```python
from build123d import *

# Parameters (mm, degrees)
F0_W         = 82.2881497443
F0_H         = 82.288146019
F0_R         = 4.2853217598
F1_DEPTH     = 25.4
F2_T1_DEPTH  = 33.02
F2_T3_DEPTH  = 107.688146019
F2_T5_DEPTH  = 72.128146019
F2_T7_DEPTH  = 72.1281497443
F2_S11_W     = 5.08
F2_S11_H     = 5.08
F2_T12_DEPTH = 5.08
F2_S17_W     = 5.08
F2_S17_H     = 5.08
F2_T18_DEPTH = 5.08
F2_S23_W     = 5.08
F2_S23_H     = 5.08
F2_T24_DEPTH = 5.08
F2_S29_W     = 5.08
F2_S29_H     = 5.08
F2_T30_DEPTH = 5.08


# Not quite as in the source:
# - a fillet or chamfer that OpenCascade refuses, or shapes differently, is made with other operations: its cross-section is extruded or revolved along the edge and cut away or added
# - a feature of the source that left no trace in its solid (it failed there, or was rolled back) is left out


with BuildPart() as f1:
    # F0 (on Front) → F1 (new body)
    with BuildSketch(Plane.XZ):
        with Locations((2.3490097374, -1.9460879266)):
            Rectangle(F0_W, F0_H)
        with Locations((-30.2557293326, 28.0709732324)):
            Circle(F0_R, mode=Mode.SUBTRACT)
        with Locations((36.1182056367, 29.1060488671)):
            Circle(F0_R, mode=Mode.SUBTRACT)
    extrude(amount=F1_DEPTH)

    # F2: fillet of radius 5.08 on 12 edges, made by hand

    # F2_s2 → F2_t1 (cut)
    with BuildSketch(Plane.XZ.offset(-12.7)):
        with BuildLine():
            ThreePointArc((38.4130846095, -43.0901609361), (42.0051870579, -41.6022633845), (43.4930846095, -38.0101609361))
            Line((43.4930846095, -38.0101609361), (43.4930846095, -43.0901609361))
            Line((43.4930846095, -43.0901609361), (38.4130846095, -43.0901609361))
        make_face()
        with BuildLine():
            ThreePointArc((38.4130846095, 39.1979850829), (42.0051870579, 37.7100875313), (43.4930846095, 34.1179850829))
            Line((43.4930846095, 34.1179850829), (43.4930846095, 39.1979850829))
            Line((43.4930846095, 39.1979850829), (38.4130846095, 39.1979850829))
        make_face()
        with BuildLine():
            ThreePointArc((-33.7150651348, 39.1979850829), (-37.3071675832, 37.7100875313), (-38.7950651348, 34.1179850829))
            Line((-38.7950651348, 34.1179850829), (-38.7950651348, 39.1979850829))
            Line((-38.7950651348, 39.1979850829), (-33.7150651348, 39.1979850829))
        make_face()
        with BuildLine():
            ThreePointArc((-38.7950651348, -38.0101609361), (-37.3071675832, -41.6022633845), (-33.7150651348, -43.0901609361))
            Line((-33.7150651348, -43.0901609361), (-38.7950651348, -43.0901609361))
            Line((-38.7950651348, -43.0901609361), (-38.7950651348, -38.0101609361))
        make_face()
    extrude(amount=F2_T1_DEPTH, mode=Mode.SUBTRACT)

    # F2_s4 → F2_t3 (cut)
    with BuildSketch(Plane.XY.offset(-55.7901609361)):
        with BuildLine():
            ThreePointArc((43.4930846095, -5.08), (42.0051870579, -1.4878975516), (38.4130846095, 0))
            Line((38.4130846095, 0), (43.4930846095, 0))
            Line((43.4930846095, 0), (43.4930846095, -5.08))
        make_face()
        with BuildLine():
            ThreePointArc((-38.7950651348, -5.08), (-37.3071675832, -1.4878975516), (-33.7150651348, 0))
            Line((-33.7150651348, 0), (-38.7950651348, 0))
            Line((-38.7950651348, 0), (-38.7950651348, -5.08))
        make_face()
    extrude(amount=F2_T3_DEPTH, mode=Mode.SUBTRACT)

    # F2_s6 → F2_t5 (cut)
    with BuildSketch(Plane.XY.offset(-38.0101609361)):
        with BuildLine():
            ThreePointArc((43.4930846095, -20.32), (42.0051870579, -23.9121024484), (38.4130846095, -25.4))
            Line((38.4130846095, -25.4), (43.4930846095, -25.4))
            Line((43.4930846095, -25.4), (43.4930846095, -20.32))
        make_face()
        with BuildLine():
            ThreePointArc((-38.7950651348, -20.32), (-37.3071675832, -23.9121024484), (-33.7150651348, -25.4))
            Line((-33.7150651348, -25.4), (-38.7950651348, -25.4))
            Line((-38.7950651348, -25.4), (-38.7950651348, -20.32))
        make_face()
    extrude(amount=F2_T5_DEPTH, mode=Mode.SUBTRACT)

    # F2_s8 → F2_t7 (cut)
    with BuildSketch(Plane.YZ.offset(-33.7150651348)):
        with BuildLine():
            ThreePointArc((-20.32, 39.1979850829), (-23.9121024484, 37.7100875313), (-25.4, 34.1179850829))
            Line((-25.4, 34.1179850829), (-25.4, 39.1979850829))
            Line((-25.4, 39.1979850829), (-20.32, 39.1979850829))
        make_face()
        with BuildLine():
            ThreePointArc((-20.32, -43.0901609361), (-23.9121024484, -41.6022633845), (-25.4, -38.0101609361))
            Line((-25.4, -38.0101609361), (-25.4, -43.0901609361))
            Line((-25.4, -43.0901609361), (-20.32, -43.0901609361))
        make_face()
    extrude(amount=F2_T7_DEPTH, mode=Mode.SUBTRACT)


with BuildPart() as f2_tool10:
    # F2_s11 → F2_t12 (new body)
    with BuildSketch(Plane.XY.offset(-38.0101609361)):
        with Locations((40.9530846095, -22.86)):
            Rectangle(F2_S11_W, F2_S11_H)
    extrude(amount=-F2_T12_DEPTH)

    # F2_s13 → F2_t14 (revolve, cut)
    with BuildSketch(Plane(origin=(38.4130846095, -20.32, -38.0101609361), x_dir=(-0.7071067812, 0.7071067812, 0), z_dir=(-0.7071067812, -0.7071067812, 0))):
        with BuildLine():
            ThreePointArc((0, -5.08), (5.08, 0), (0, 5.08))
            Line((0, 5.08), (0, -5.08))
        make_face()
    revolve(axis=Axis((38.4130846095, -20.32, -38.0101609361), (0, 0, -1)), mode=Mode.SUBTRACT)


with BuildPart() as f1_1:
    add(f1.part)

    # F2_t9: cut F2_tool10
    add(f2_tool10.part, mode=Mode.SUBTRACT)


with BuildPart() as f2_tool16:
    # F2_s17 → F2_t18 (new body)
    with BuildSketch(Plane.XY.offset(34.1179850829)):
        with Locations((40.9530846095, -22.86)):
            Rectangle(F2_S17_W, F2_S17_H)
    extrude(amount=F2_T18_DEPTH)

    # F2_s19 → F2_t20 (revolve, cut)
    with BuildSketch(Plane(origin=(38.4130846095, -20.32, 34.1179850829), x_dir=(-0.7071067812, 0.7071067812, 0), z_dir=(0.7071067812, 0.7071067812, 0))):
        with BuildLine():
            ThreePointArc((0, -5.08), (5.08, 0), (0, 5.08))
            Line((0, 5.08), (0, -5.08))
        make_face()
    revolve(axis=Axis((38.4130846095, -20.32, 34.1179850829), (0, 0, 1)), mode=Mode.SUBTRACT)


with BuildPart() as f1_2:
    add(f1_1.part)

    # F2_t15: cut F2_tool16
    add(f2_tool16.part, mode=Mode.SUBTRACT)


with BuildPart() as f2_tool22:
    # F2_s23 → F2_t24 (new body)
    with BuildSketch(Plane.XY.offset(34.1179850829)):
        with Locations((-36.2550651348, -22.86)):
            Rectangle(F2_S23_W, F2_S23_H)
    extrude(amount=F2_T24_DEPTH)

    # F2_s25 → F2_t26 (revolve, cut)
    with BuildSketch(Plane(origin=(-33.7150651348, -20.32, 34.1179850829), x_dir=(0.7071067812, 0.7071067812, 0), z_dir=(0.7071067812, -0.7071067812, 0))):
        with BuildLine():
            ThreePointArc((0, -5.08), (5.08, 0), (0, 5.08))
            Line((0, 5.08), (0, -5.08))
        make_face()
    revolve(axis=Axis((-33.7150651348, -20.32, 34.1179850829), (0, 0, 1)), mode=Mode.SUBTRACT)


with BuildPart() as f1_3:
    add(f1_2.part)

    # F2_t21: cut F2_tool22
    add(f2_tool22.part, mode=Mode.SUBTRACT)


with BuildPart() as f2_tool28:
    # F2_s29 → F2_t30 (new body)
    with BuildSketch(Plane.YZ.offset(-33.7150651348)):
        with Locations((-22.86, -40.5501609361)):
            Rectangle(F2_S29_W, F2_S29_H)
    extrude(amount=-F2_T30_DEPTH)

    # F2_s31 → F2_t32 (revolve, cut)
    with BuildSketch(Plane(origin=(-33.7150651348, -20.32, -38.0101609361), x_dir=(0, 0.7071067812, 0.7071067812), z_dir=(0, -0.7071067812, 0.7071067812))):
        with BuildLine():
            ThreePointArc((0, -5.08), (5.08, 0), (0, 5.08))
            Line((0, 5.08), (0, -5.08))
        make_face()
    revolve(axis=Axis((-33.7150651348, -20.32, -38.0101609361), (-1, 0, 0)), mode=Mode.SUBTRACT)


with BuildPart() as f1_4:
    add(f1_3.part)

    # F2_t27: cut F2_tool28
    add(f2_tool28.part, mode=Mode.SUBTRACT)

    # F2_s33 → F2_t34 (revolve, cut)
    with BuildSketch(Plane.XY.offset(28.0709732324)):
        with BuildLine():
            ThreePointArc((-25.9704075728, -20.32), (-24.4825100212, -23.9121024484), (-20.8904075728, -25.4))
            Line((-20.8904075728, -25.4), (-25.9704075728, -25.4))
            Line((-25.9704075728, -25.4), (-25.9704075728, -20.32))
        make_face()
    revolve(axis=Axis((-30.2557293326, -25.4, 28.0709732324), (0, -1, 0)), mode=Mode.SUBTRACT)

    # F2_s35 → F2_t36 (revolve, cut)
    with BuildSketch(Plane.XY.offset(29.1060488671)):
        with BuildLine():
            ThreePointArc((40.4035273965, -20.32), (41.8914249481, -23.9121024484), (45.4835273965, -25.4))
            Line((45.4835273965, -25.4), (40.4035273965, -25.4))
            Line((40.4035273965, -25.4), (40.4035273965, -20.32))
        make_face()
    revolve(axis=Axis((36.1182056367, -25.4, 29.1060488671), (0, -1, 0)), mode=Mode.SUBTRACT)


solid = f1_4.part
```
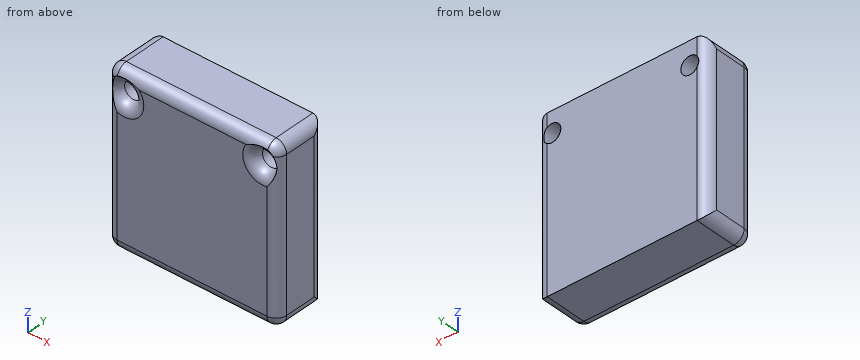
Work out the finished part from the listing and answer in its coordinate system (mm). Round coordinates to 2 decimals unless told otherwise and drop trailing zeros. Order: outer loops, then holes, each group sorted by start corner. A loop starts at its lowest first (then second) coordinate and runs counter-clockwise, first axis right, second up.
Q1. Find the intervals of material crossed by line 1 along X through (y, z) = (-13.25, 29); line 2 along X through (y, z) = (-7, 24.5); line 3 along X through (y, z) = (-5, -19.5), in increasing order.
Solution:
line 1: x = -38.8 to -34.44, -26.07 to 31.83, 40.4 to 43.49
line 2: x = -38.8 to -32.62, -27.89 to 43.49
line 3: x = -38.79 to 43.49
Q2. A cutting plane is placed at B-B, the plane y = -21.75. Determine the outline of the cut face in (x, z).
Solution:
outline: (-38.59, -38.01) arc R4.87 ccw to (-33.72, -42.88) - (38.41, -42.88) arc R4.87 ccw to (43.29, -38.01) - (43.29, 34.12) arc R4.87 ccw to (38.41, 38.99) - (-33.72, 38.99) arc R4.87 ccw to (-38.59, 34.12) - close; hole circle Ø8.98 at (-30.26, 28.07); hole circle Ø8.98 at (36.12, 29.11)
Q3. A cutting plane is placed at A-A, the plane y = -2. Determine the outline of the cut face in (x, z).
Solution:
outline: (-37.75, -41.09) arc R5.08 ccw to (-33.72, -43.09) - (38.41, -43.09) arc R5.08 ccw to (42.45, -41.09) - (42.45, 37.2) arc R5.08 ccw to (38.41, 39.2) - (-33.72, 39.2) arc R5.08 ccw to (-37.75, 37.2) - close; hole circle Ø8.57 at (-30.26, 28.07); hole circle Ø8.57 at (36.12, 29.11)
Q4. Given pin 1 Ø5 at (x, z) = (-30.26, 28.07) entering from +Y; pin 2 Ø10 at (x, z) = (36.12, 29.11) entering from -Y, each flat-ended and moving along its own axis, determine where each tip first touches the part or whether it passes through.
Solution:
pin 1: passes through
pin 2: stops at y = -22.93
